Check sheet for the drawn part. Datum: minimum x, y, z corner. Units: mm. A direction names the side the tool comes from. Round coordinates to 2 decimals unless told otherwise and drop trailing zeros. Write each loop counter-clockwise with the first axis right and the second up, starting at its lowest first coordinate (ties: lowest second). Pieces come first, ordered by that corner, then holes. Notation, with made-up numbers: M 87,-37 L 141,-37 A32 ccw 141,-10 Z; hole C -36,79 d2. An arc over 180 degrees is marked long. One line per item, written item: value. Start each with the question number.
Item 1: Section check A-A, the plane y = 6.5. Record the cut outline in (x, z), then the cut area to 3 significant figures.
Item 2: Section check B-B, the plane x = 7. Record the cut outline in (y, z), then the cut area to 3 significant figures.
Item 3: Section check C-C, the plane z = 4.5. Record the cut outline in (x, y), then the cut area to 3 significant figures.
Item 4: Gauge pin test, flat ends, axial feed: pin 1 (3 mm diameter, centred on y = 8.5, z = 4.5, fed in from -X); pin 2 (4 mm diameter, centred on x = 6.5, y = 6.5, fed in from +Z); pin 3 (1 mm diameter, centred on x = 9, z = 4.5, fed in from +Y); pin 4 (3 mm diameter, centred on y = 10.5, z = 8, fed in from +X). Record the tip position at first contact, or that the pin passes through.
Item 5: Section check D-D, the plane y = 3.5. Record the cut outline in (x, z).
Item 6: Thickness scan on probe 1 along X at (y, z) = (6.5, 4.65); probe 2 along X at (y, z) = (6.5, 1). Record the ranges inside material, lowest first. Write a range as from..to.
Item 7: Tool access check on the marked faces 1, 2, 3, 4 and 5. Record the directions out of +Z, -Z, +X, -X, +Y, -Y that give a thin tool (end or side, any length) a straight path to the whole face; none if there is none.
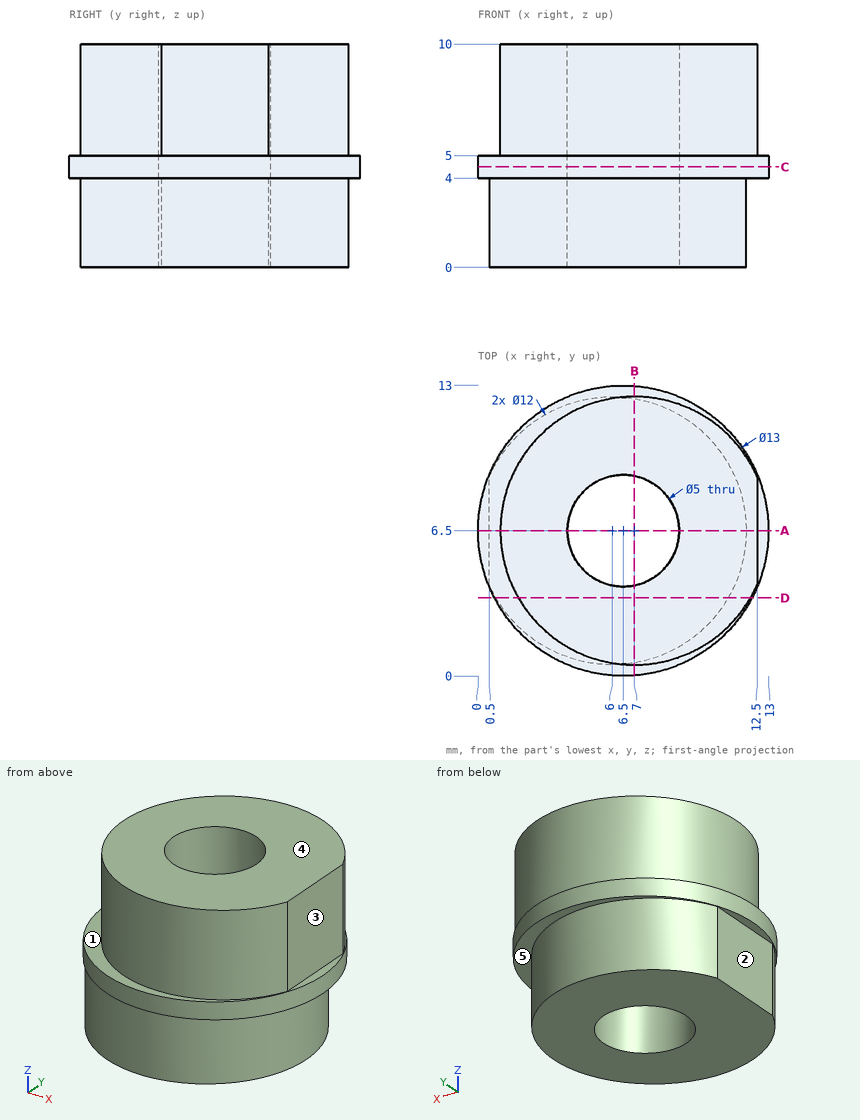
Response values:
1. outline: M 0,4 L 0.5,4 L 0.5,0 L 4,0 L 4,10 L 1,10 L 1,5 L 0,5 Z; M 9,0 L 12,0 L 12,4 L 13,4 L 13,5 L 12.5,5 L 12.5,10 L 9,10 Z
1. area: 66.5 mm2
2. outline: M 0.02,4 L 0.58,4 L 0.58,0 L 4.05,0 L 4.05,10 L 0.5,10 L 0.5,5 L 0.02,5 Z; M 8.95,0 L 12.42,0 L 12.42,4 L 12.98,4 L 12.98,5 L 12.5,5 L 12.5,10 L 8.95,10 Z
2. area: 71.3 mm2
3. outline: C 6.5,6.5 d13; hole C 6.5,6.5 d5
3. area: 113 mm2
4. pin 1: stops at x = 0.02
4. pin 2: passes through
4. pin 3: stops at y = 12.68
4. pin 4: stops at x = 12.45
5. outline: M 0.73,4 L 0.8,4 L 0.8,0 L 11.2,0 L 11.2,4 L 12.27,4 L 12.27,5 L 12.2,5 L 12.2,10 L 1.8,10 L 1.8,5 L 0.73,5 Z
6. probe 1: x = 0..4, 9..13
6. probe 2: x = 0.5..4, 9..12
7. face 1: +Z
7. face 2: -Z, -X, +Y, -Y
7. face 3: +Z, +X, +Y, -Y
7. face 4: +Z, +X, -X, +Y, -Y
7. face 5: -Z
